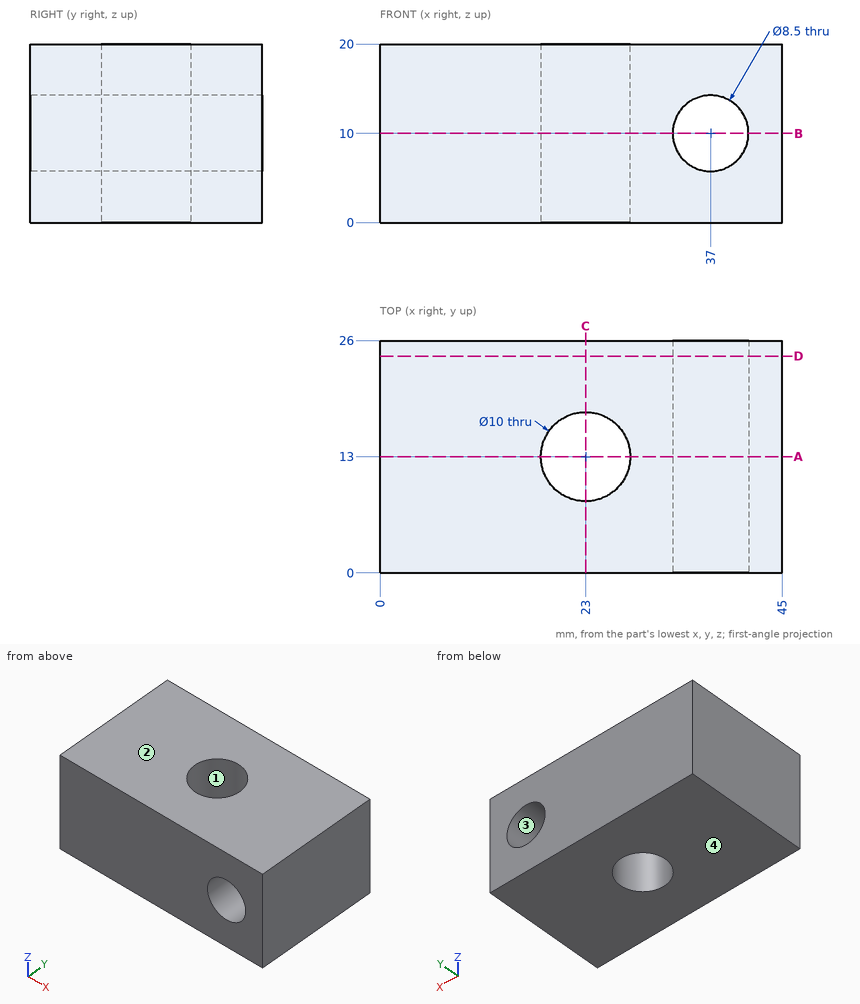
Input: dimensioned drawing with shaded views. Units: mm. Origin: part minimum x, y, z. Coordinates: 2 decimals unless noted, no trailing zeros. Write each loop counter-clockwise with the first axis right and the second up, starting at its lowest first coordinate (ties: lowest second). Pieces come first, ordered by that corner, then holes. Notation, with made-up numbers: M 35,-4 L 61,-4 A25 cw 61,10 Z; hole C 66,-30.75 d3. An arc over 180 degrees is marked long. Use one line per item in the form item = value.
Q1. Section D-D (y = 24.25). Return loops of the section in (x, z).
Answer below:
outline = M 0,0 L 45,0 L 45,20 L 0,20 Z; hole C 37,10 d8.5
Q2. Material intervals for probe 1 along Y at (x, z) = (23, 15.5); probe 2 along Z at (x, y) = (37, 12.25); probe 3 along X at (y, z) = (13, 12.5), sorted ascending. Write a range as from..to.
Answer below:
probe_1 = 0..8, 18..26
probe_2 = 0..5.75, 14.25..20
probe_3 = 0..18, 28..33.56, 40.44..45
Q3. Section C-C (x = 23). Return loops of the section in (y, z), plus the area to 3 significant figures.
Answer below:
outline = M 0,0 L 8,0 L 8,20 L 0,20 Z; M 18,0 L 26,0 L 26,20 L 18,20 Z
area = 320 mm²
Q4. Draft query along Z for the marked faces 1, 2, 3 and 4. Return one class per face: released by +Z, released by -Z, zero draft, split by the parting line, or undercut.
Answer below:
face_1 = zero draft
face_2 = released by +Z
face_3 = undercut
face_4 = released by -Z
Q5. Section B-B (z = 10). Return loops of the section in (x, y), plus the area to 3 significant figures.
Answer below:
outline = M 0,0 L 32.75,0 L 32.75,26 L 0,26 Z; M 41.25,0 L 45,0 L 45,26 L 41.25,26 Z; hole C 23,13 d10
area = 870 mm²
Q6. Section A-A (y = 13). Return loops of the section in (x, z).
Answer below:
outline = M 0,0 L 18,0 L 18,20 L 0,20 Z; M 28,0 L 45,0 L 45,20 L 28,20 Z; hole C 37,10 d8.5
